The listing builds one solid part. Answer for the finished solid, in the listing's coordinates (mm). A direction names the side the tool comes from. Round coordinates to 2 decimals unless told otherwise and drop trailing zeros. Write each loop counter-clockwise with the first axis right and the second up, starting at its lowest first coordinate (ties: lowest second). Pieces come first, ordered by that corner, then holes. Notation, with made-up numbers: M 17.25,84.5 L 33.25,84.5 A9 ccw 33.25,96.5 Z; hole C -2.75,61 d10. An arc over 180 degrees is marked long. Write each question's results on one line, items separated by ' | '.
from build123d import *

# Parameters (mm, degrees)
BOSS_EXTRUDE1_DEPTH = 5
SKETCH5_R           = 5
CUT_EXTRUDE4_DEPTH  = 5
SKETCH2_R           = 5
CUT_EXTRUDE5_DEPTH  = 5
BOSS_EXTRUDE2_DEPTH = 5


with BuildPart() as part:
    # Sketch1 → Boss-Extrude1 (new body)
    with BuildSketch(Plane(origin=(0, 0, 0), x_dir=(0, 0, -1), z_dir=(1, 0, 0))):
        Polygon((-75, 70), (-120, 70), (-120, 55), (-130, 55), (-130, 15), (-120, 15), (-120, 0), (-75, 0), (-75, 5), (-35, 5), (-35, 0), (-10, 0), (0, 0), (0, 15), (0, 55), (0, 70), (-10, 70), (-35, 70), (-35, 60), (-75, 60), align=None)
    extrude(amount=BOSS_EXTRUDE1_DEPTH)

    # Sketch5 → Cut-Extrude4 (cut)
    with BuildSketch(Plane.ZY):
        with Locations((17.111667647, 26.5)):
            Circle(SKETCH5_R)
        with Locations((52.52, 33)):
            Circle(SKETCH5_R)
    extrude(amount=-CUT_EXTRUDE4_DEPTH, mode=Mode.SUBTRACT)

    # Sketch2 → Cut-Extrude5 (cut)
    with BuildSketch(Plane(origin=(5, 0, 0), x_dir=(0, 0, -1), z_dir=(1, 0, 0))):
        with Locations((-88.52, 40)):
            Circle(SKETCH2_R)
    extrude(amount=-CUT_EXTRUDE5_DEPTH, mode=Mode.SUBTRACT)

    # Sketch6 → Boss-Extrude2 (add)
    with BuildSketch(Plane.ZY):
        Polygon((35, 0), (35, 5), (75, 5), (75, 0), (120, 0), (120, 15), (130, 15), (130, 55), (120, 55), (120, 70), (75, 70), (75, 60), (35, 60), (35, 70), (0, 70), (0, 0), align=None)
    extrude(amount=BOSS_EXTRUDE2_DEPTH)


solid = part.part
1) The mould has two halves that part along Z. Classify faces 6 (the face through (5, 35, 66)), 7 (the face through (0, 62, 120)), 8 (the face through (2.465, 22.064, 19.419)): +Z half, -Z half, draft (parallel to the pull), parting line (faces both ways), or undercut.
Return value:
face 6: draft | face 7: +Z half | face 8: undercut
2) Section B-B (x = 1.25) is taken. Determine the outline of the cut face in (y, z).
Return value:
outline: M 0,0 L 70,0 L 70,35 L 60,35 L 60,75 L 70,75 L 70,120 L 55,120 L 55,130 L 15,130 L 15,120 L 0,120 L 0,75 L 5,75 L 5,35 L 0,35 Z; hole C 26.5,17.11 d10; hole C 33,52.52 d10; hole C 40,88.52 d10
3) Section C-C (y = 40) is taken. Determine the outline of the cut face in (x, z).
Return value:
outline: M -5,0 L 5,0 L 5,83.52 L 0,83.52 L 0,93.52 L 5,93.52 L 5,130 L -5,130 Z
4) A tool of negligible diameter and unlimited length cuts with its end or side. For faces 1 (the face through (0, 15, 125)), 2 (the face through (0, 55, 125)), 3 (the face through (0, 3, 75)), 4 (the face through (0, 60, 55)), 5 (the face through (0, 27, 17)), from which of +Z, -Z, +X, -X, +Y, -Y can it reach the whole face along a straight path? Write none if from no direction.
Return value:
face 1: +Z, +X, -X, -Y | face 2: +Z, +X, -X, +Y | face 3: +X, -X, -Y | face 4: +X, -X, +Y | face 5: +X
5) Each of these flat-tipped pins is pushed along its axis until it touches: pin 1 (5 mm diameter, centred on x = -1.5, y = 6.5, fed in from +Z); pin 2 (3 mm diameter, centred on x = -1, z = 57, fed in from +Y); pin 3 (3 mm diameter, centred on x = 0, z = 124, fed in from +Y). Where does it stop, or does it pass through?
Return value:
pin 1: z = 120 | pin 2: y = 60 | pin 3: y = 55
6) Section A-A (y = 62.5) is taken. Determine the outline of the cut face in (x, z).
Return value:
outline: M -5,0 L 5,0 L 5,35 L -5,35 Z; M -5,75 L 5,75 L 5,120 L -5,120 Z
7) Find the intervals of material crossed by line 1 (Y direction, x = 2.6, z = 88.52); line 2 (Y direction, x = 2.45, z = 52.52); line 3 (Z direction, x = -0.25, y = 4.5), in increasing order.
Return value:
line 1: 0 to 35, 45 to 70 | line 2: 5 to 28, 38 to 60 | line 3: 0 to 35, 75 to 120
8) Section D-D (z = 52.52) is taken. Determine the outline of the cut face in (x, y).
Return value:
outline: M -5,5 L 5,5 L 5,28 L 0,28 L 0,38 L 5,38 L 5,60 L -5,60 Z
